Work out the finished part from the listing and answer in its coordinate system (mm). Face numbers are marked on the shaded views. A direction names the side the tool comes from. Coordinates: 2 decimals unless noted, no trailing zeros. Order: outer loops, then holes, each group sorted by start corner. A loop starts at its lowest first (then second) coordinate and runs counter-clockwise, first axis right, second up. Notation, with made-up numbers: (11, -8.75) -> (22, -8.75) arc R28 ccw to (22, 13.25) -> close; hole circle Ø6 at (85.5, 75). An arc over 180 degrees is marked (long way). Answer as CSV lines item,"result". Start each with the question number.
Item 1: Section C-C (z = 5) is taken. Write down the section's boundary in (x, y), then the cut area to 3 significant figures.
Item 2: Each of these flat-tipped pins is pushed along its axis until it touches: pin 1 Ø1.9 at (x, z) = (15.5, 18.5) entering from -Y; pin 2 Ø2 at (x, y) = (16, -4.5) entering from +Z; pin 3 Ø3 at (x, y) = (6.5, -177) entering from -Z. Where does it stop, or does it pass through?
Item 3: Straight lines are drawn through the part: L1, parallel to Y at x = 6.25, z = 16; L2, parallel to Z at x = 24, y = -55; L3, parallel to Y at x = 7.75, z = 19.5. For each, find the intervals that lie inside material, in ascending order.
Item 4: Section A-A (x = 10) is taken. Write down the section's boundary in (y, z).
Item 5: Section B-B (y = -145) is taken. Write down the section's boundary in (x, z).
Item 6: Section D-D (z = 32) is taken. Write down the section's boundary in (x, y), then the cut area to 3 significant figures.
Item 7: Which of the six approach directions +Z, -Z, +X, -X, +Y, -Y give full straight-line access (tool end or side, diameter ignored) to the marked faces 1 and 2?
```python
from build123d import *

# Parameters (mm, degrees)
F0_W          = 88.9
F0_H          = 1.905
F1_DEPTH      = 25.4
F2_W          = 12.7
F2_H          = 88.9715382425
F2_H_2        = 50.7284617575
F3_DEPTH      = 50.8
F3_DEPTH_BACK = 25.4
F4_W          = 6.35
F4_H          = 3.81
F5_DEPTH      = 2.54
F6_W          = 12.7
F6_H          = 12.7
F7_DEPTH      = 7.62
F9_DEPTH      = 25.4


with BuildPart() as f1:
    # F0 (on Right) → F1 (new body)
    with BuildSketch(Plane.YZ):
        with Locations((14.6420187533, 19.2617916149)):
            Rectangle(F0_W, F0_H)
        with Locations((14.6420187533, 17.3567916149)):
            Rectangle(F0_W, F0_H)
        with BuildLine():
            ThreePointArc((-29.8795194892, 20.2142916149), (-29.8258721082, 19.2624629951), (-29.8079812467, 18.3092916149))
            Line((-29.8079812467, 18.3092916149), (-29.8079812467, 20.2142916149))
            Line((-29.8079812467, 20.2142916149), (-29.8795194892, 20.2142916149))
        make_face()
        with BuildLine():
            Line((-29.8079812467, 16.4042916149), (-29.8079812467, 18.3092916149))
            ThreePointArc((-29.8079812467, 18.3092916149), (-29.8258721082, 17.3561202347), (-29.8795194892, 16.4042916149))
            Line((-29.8795194892, 16.4042916149), (-29.8079812467, 16.4042916149))
        make_face()
        with BuildLine():
            ThreePointArc((-29.8795194892, 16.4042916149), (-29.8258721082, 17.3561202347), (-29.8079812467, 18.3092916149))
            ThreePointArc((-29.8079812467, 18.3092916149), (-29.8258721082, 19.2624629951), (-29.8795194892, 20.2142916149))
            Line((-29.8795194892, 20.2142916149), (-36.2534705698, 20.2142916149))
            ThreePointArc((-36.2534705698, 20.2142916149), (-36.181868554, 19.2629874798), (-36.1579812467, 18.3092916149))
            ThreePointArc((-36.1579812467, 18.3092916149), (-36.181868554, 17.35559575), (-36.2534705698, 16.4042916149))
            Line((-36.2534705698, 16.4042916149), (-29.8795194892, 16.4042916149))
        make_face()
        with BuildLine():
            Line((-36.2534705698, 20.2142916149), (-29.8795194892, 20.2142916149))
            ThreePointArc((-29.8795194892, 20.2142916149), (-55.2079812467, 43.7092916149), (-80.5364430042, 20.2142916149))
            Line((-80.5364430042, 20.2142916149), (-74.1624919236, 20.2142916149))
            ThreePointArc((-74.1624919236, 20.2142916149), (-55.2079812467, 37.3592916149), (-36.2534705698, 20.2142916149))
        make_face()
        with BuildLine():
            ThreePointArc((-80.5364430042, 16.4042916149), (-55.2079812467, -7.0907083851), (-29.8795194892, 16.4042916149))
            Line((-29.8795194892, 16.4042916149), (-36.2534705698, 16.4042916149))
            ThreePointArc((-36.2534705698, 16.4042916149), (-55.2079812467, -0.7407083851), (-74.1624919236, 16.4042916149))
            Line((-74.1624919236, 16.4042916149), (-80.5364430042, 16.4042916149))
        make_face()
        with BuildLine():
            Line((-74.1624919236, 20.2142916149), (-80.5364430042, 20.2142916149))
            ThreePointArc((-80.5364430042, 20.2142916149), (-80.6079812467, 18.3092916149), (-80.5364430042, 16.4042916149))
            Line((-80.5364430042, 16.4042916149), (-74.1624919236, 16.4042916149))
            ThreePointArc((-74.1624919236, 16.4042916149), (-74.2579812467, 18.3092916149), (-74.1624919236, 20.2142916149))
        make_face()
        with BuildLine():
            ThreePointArc((-80.5364430042, 16.4042916149), (-80.6079812467, 18.3092916149), (-80.5364430042, 20.2142916149))
            Line((-80.5364430042, 20.2142916149), (-169.5079812467, 20.2142916149))
            Line((-169.5079812467, 20.2142916149), (-169.5079812467, 16.4042916149))
            Line((-169.5079812467, 16.4042916149), (-80.5364430042, 16.4042916149))
        make_face()
    extrude(amount=F1_DEPTH)

    # F2 (on face) → F3 (cut, two sides)
    with BuildSketch(Plane.XY.offset(20.2142916149)) as f3_sk:
        with Locations((12.7, -125.0222121254)):
            Rectangle(F2_W, F2_H)
        with Locations((12.7, -55.1722121254)):
            Rectangle(F2_W, F2_H_2)
    extrude(amount=-F3_DEPTH, mode=Mode.SUBTRACT)
    extrude(f3_sk.sketch, amount=F3_DEPTH_BACK, mode=Mode.SUBTRACT)

    # F4 (on face) → F5 (join)
    with BuildSketch(Plane.XZ.offset(169.5079812467)):
        Polygon((25.4, 20.2142916149), (6.35, 20.2142916149), (6.35, 16.4042916149), (0, 16.4042916149), (0, -5.1857083851), (25.4, -5.1857083851), align=None)
        with Locations((3.175, 18.3092916149)):
            Rectangle(F4_W, F4_H)
    extrude(amount=F5_DEPTH)

    # F6 (on face) → F7 (join)
    with BuildSketch(Plane.XZ.offset(172.0479812467)):
        with Locations((12.7, 1.1642916149)):
            Rectangle(F6_W, F6_H)
    extrude(amount=F7_DEPTH)

    # F8 (on face) → F9 (cut)
    with BuildSketch(Plane.YZ.offset(19.05)):
        Polygon((-179.6679812467, 7.5142916149), (-179.6679812467, -5.1857083851), (-172.0479812467, 7.5142916149), align=None)
    extrude(amount=-F9_DEPTH, mode=Mode.SUBTRACT)


solid = f1.part
```
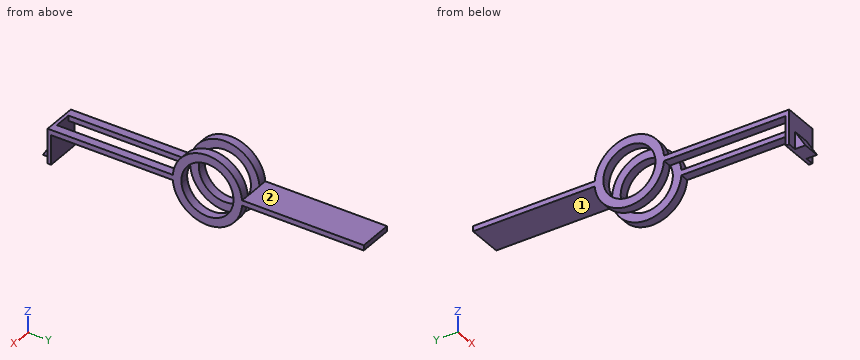
Checked values:
1,outline,"(0, -172.05) -> (6.35, -172.05) -> (6.35, -173.56) -> (19.05, -173.56) -> (19.05, -172.05) -> (25.4, -172.05) -> (25.4, -169.51) -> (0, -169.51) -> close; (0, -76.84) -> (6.35, -76.84) -> (6.35, -68.84) -> (0, -68.84) -> close; (0, -41.58) -> (6.35, -41.58) -> (6.35, -33.57) -> (0, -33.57) -> close; (19.05, -76.84) -> (25.4, -76.84) -> (25.4, -68.84) -> (19.05, -68.84) -> close; (19.05, -41.58) -> (25.4, -41.58) -> (25.4, -33.57) -> (19.05, -33.57) -> close"
1,area,"287 mm^2"
2,pin 1,"stops at y = -172.05"
2,pin 2,"stops at z = 20.21"
2,pin 3,"stops at z = -5.19"
3,L1,"y = -172.05 to -169.51, -80.5 to -74.12, -36.3 to -29.91"
3,L2,"z = -7.09 to -0.74, 37.36 to 43.71"
3,L3,"y = -172.05 to -169.51, -29.81 to 59.09"
4,outline,"(-179.67, -5.19) -> (-169.51, -5.19) -> (-169.51, 20.21) -> (-172.05, 20.21) -> (-172.05, 7.51) -> close; (-29.81, 16.4) -> (59.09, 16.4) -> (59.09, 20.21) -> (-29.81, 20.21) -> close"
5,outline,"(0, 16.4) -> (6.35, 16.4) -> (6.35, 20.21) -> (0, 20.21) -> close; (19.05, 16.4) -> (25.4, 16.4) -> (25.4, 20.21) -> (19.05, 20.21) -> close"
6,outline,"(0, -76.6) -> (6.35, -76.6) -> (6.35, -68.45) -> (0, -68.45) -> close; (0, -41.96) -> (6.35, -41.96) -> (6.35, -33.81) -> (0, -33.81) -> close; (19.05, -76.6) -> (25.4, -76.6) -> (25.4, -68.45) -> (19.05, -68.45) -> close; (19.05, -41.96) -> (25.4, -41.96) -> (25.4, -33.81) -> (19.05, -33.81) -> close"
6,area,"207 mm^2"
7,face 1,"-Z, +X, -X, +Y"
7,face 2,"+Z, +X, -X, +Y"
